Build history of the part. All positions in model axes, mm. Round coordinates to 2 decimals unless told otherwise and drop trailing zeros.
Item 1: Wall check: probe 1 along Y at (x, z) = (172, 0); probe 2 along Y at (x, z) = (104.5, -1.25); probe 3 along X at (y, z) = (28, -0.5). Give the ranges that are in metal, low to high.
Item 2: Mould opens along Y. For faces 1 (the flat face through (106, -1, 1)), 2 (the flat face through (105, 17, -2)) say: +Y half, -Y half, draft (parallel to the pull), parting line (faces both ways), or undercut.
Item 3: Drop flat-ended pins along their axis: pin 1 Ø4 at (y, z) = (27.5, -11.5) entering from -X; pin 2 Ø2 at (x, y) = (126.5, 2) entering from +Z; pin 3 Ø0.9 at (x, z) = (126, 0) entering from +Y. Give the stop position or say it passes through.
```python
from build123d import *

# Parameters (mm, degrees)
F0_W          = 217
F0_H          = 38
F0_W_2        = 213
F0_H_2        = 34
F1_DEPTH      = 1
F2_DEPTH      = 17
F2_TAPER      = -45
F3_DEPTH      = 2
F5_DEPTH      = 53.0010001
F5_DEPTH_BACK = 25


with BuildPart() as f1:
    # F0 (on Top) → F1 (new body)
    with BuildSketch(Plane.XY):
        with Locations((106.5, 17)):
            Rectangle(F0_W, F0_H)
        with Locations((106.5, 17)):
            Rectangle(F0_W_2, F0_H_2, mode=Mode.SUBTRACT)
    extrude(amount=F1_DEPTH)

    # F0 (on Top) → F2 (join)
    with BuildSketch(Plane.XY):
        with Locations((106.5, 17)):
            Rectangle(F0_W, F0_H)
        with Locations((106.5, 17)):
            Rectangle(F0_W_2, F0_H_2, mode=Mode.SUBTRACT)
        with Locations((106.5, 17)):
            Rectangle(F0_W_2, F0_H_2)
    extrude(amount=-F2_DEPTH, taper=F2_TAPER)

    # F0 (on Top) → F3 (cut)
    with BuildSketch(Plane.XY):
        with Locations((106.5, 17)):
            Rectangle(F0_W_2, F0_H_2)
    extrude(amount=-F3_DEPTH, mode=Mode.SUBTRACT)

    # F4 (on Front) → F5 (cut, two sides)
    with BuildSketch(Plane.XZ) as f5_sk:
        Polygon((217.1184106235, -2.1184106235), (-19, -17), (234.9526717854, -19.9526717854), align=None)
    extrude(amount=-F5_DEPTH, mode=Mode.SUBTRACT)
    extrude(f5_sk.sketch, amount=F5_DEPTH_BACK, mode=Mode.SUBTRACT)


solid = f1.part
```
Results:
1. probe 1: y = -2 to 0, 34 to 36
1. probe 2: y = -3.25 to 0, 34 to 37.25
1. probe 3: x = -2.5 to 0, 213 to 215.5
2. face 1: draft
2. face 2: undercut
3. pin 1: stops at x = -15.5
3. pin 2: stops at z = -2
3. pin 3: stops at y = 36.45
